from build123d import *

# Parameters (mm, degrees)
SKETCH1_W           = 25
SKETCH1_H           = 50
BOSS_EXTRUDE1_DEPTH = 4.5
CUT_EXTRUDE2_REACH  = 6.5


with BuildPart() as part:
    # Sketch1 → Boss-Extrude1 (new body)
    with BuildSketch(Plane.XY):
        with Locations((12.5, 25)):
            Rectangle(SKETCH1_W, SKETCH1_H)
    extrude(amount=BOSS_EXTRUDE1_DEPTH)

    # Sketch3 → Cut-Extrude2 (cut, up to next)
    with BuildSketch(Plane.XY.offset(4.5), mode=Mode.PRIVATE) as cut_extrude2_sk1:
        with BuildLine():
            Line((6.5, 18.25), (18.5, 18.25))
            ThreePointArc((18.5, 18.25), (18.886370331, 17.953527618), (18.7, 17.503589838))
            ThreePointArc((18.7, 17.503589838), (18.553589838, 17.357179677), (18.5, 17.157179677))
            Line((18.5, 17.157179677), (18.5, 14.842820323))
            ThreePointArc((18.5, 14.842820323), (18.553589838, 14.642820323), (18.7, 14.496410162))
            ThreePointArc((18.7, 14.496410162), (18.886370331, 14.046472382), (18.5, 13.75))
            Line((18.5, 13.75), (6.5, 13.75))
            ThreePointArc((6.5, 13.75), (6.113629669, 14.046472382), (6.3, 14.496410162))
            ThreePointArc((6.3, 14.496410162), (6.446410162, 14.642820323), (6.5, 14.842820323))
            Line((6.5, 14.842820323), (6.5, 17.157179677))
            ThreePointArc((6.5, 17.157179677), (6.446410162, 17.357179677), (6.3, 17.503589838))
            ThreePointArc((6.3, 17.503589838), (6.113629669, 17.953527618), (6.5, 18.25))
        make_face()
    cut_extrude2_tool1 = extrude(cut_extrude2_sk1.sketch, amount=-CUT_EXTRUDE2_REACH, mode=Mode.PRIVATE) & part.part
    add(cut_extrude2_tool1.solids().sort_by_distance((12.5, 16, 4.5))[0], mode=Mode.SUBTRACT)


solid = part.part
Verification items for the finished model (mm, model axes). A direction names the side the tool comes from. Give positions to 0.01 mm unless a question says otherwise; leave off trailing zeros. Write each loop counter-clockwise with the first axis right and the second up, starting at its lowest first coordinate (ties: lowest second). Pieces come first, ordered by that corner, then holes.
(1) Mould release check, pull along X, two halves, no side actions. Record for faces 1 (the face through (13, 13.75, 2)), 2 (the face through (12, 0, 2)), 3 (the face through (18.5, 16, 2)), 4 (the face through (0, 25, 2)): +X half, -X half, draft (parallel to the pull), parting line (faces both ways), or undercut.
(2) Gauge pin test, flat end, axial feed: pin 1 (1.9 mm diameter, centred on y = 15.5, z = 2, fed in from -X). Record the tip position at first contact, or that the pin passes through.
(3) Material ranges on line 1 (Y direction, x = 17, z = 2.1); line 2 (X direction, y = 14, z = 2.7), recorded low to high.
(4) Access from +Z, -Z, +X, -X, +Y, -Y to the whole of each face (thin tool, end or side, straight path). Record for faces 5 (the face through (12, 18.25, 2)), 6 (the face through (25, 25, 2)).
(5) Cross-section at A-A (x = 16.5). Enter the section's corners in (y, z), plus the area to 3 significant figures.
(6) Cross-section at B-B (z = 1.55). Enter the section's corners in (x, y).
Worked out:
1. face 1: undercut
1. face 2: draft
1. face 3: undercut
1. face 4: -X half
2. pin 1: stops at x = 0
3. line 1: y = 0 to 13.75, 18.25 to 50
3. line 2: x = 0 to 6.13, 18.87 to 25
4. face 5: +Z, -Z
4. face 6: +Z, -Z, +X, +Y, -Y
5. outline: (0, 0) - (13.75, 0) - (13.75, 4.5) - (0, 4.5) - close; (18.25, 0) - (50, 0) - (50, 4.5) - (18.25, 4.5) - close
5. area: 205 mm2
6. outline: (0, 0) - (25, 0) - (25, 50) - (0, 50) - close; hole (6.3, 14.5) arc R0.4 ccw to (6.5, 13.75) - (18.5, 13.75) arc R0.4 ccw to (18.7, 14.5) arc R0.4 cw to (18.5, 14.84) - (18.5, 17.16) arc R0.4 cw to (18.7, 17.5) arc R0.4 ccw to (18.5, 18.25) - (6.5, 18.25) arc R0.4 ccw to (6.3, 17.5) arc R0.4 cw to (6.5, 17.16) - (6.5, 14.84) arc R0.4 cw to start
